Study the drawing (mm; zero at the part's minimum x, y, z) and answer. A direction names the side the tool comes from. Round coordinates to 2 decimals unless told otherwise and drop trailing zeros. Write each loop counter-clockwise with the first axis right and the second up, starting at its lowest first coordinate (ties: lowest second). Pieces come first, ordered by that corner, then holes. Notation, with made-up numbers: (-39, -7.5) - (-9, -7.5) arc R14 ccw to (-9, 4.5) - close; hole circle Ø5 at (23, 80). An arc over 180 degrees is marked (long way). Return JSON: item names as keys, results as strings. Group by question number.
(1) Section B-B, the plane z = 3 is taken. Write down the section's boundary in (x, y), then the cut area to 3 significant figures.
(2) Find the intervals of material crossed by line 1 along X through (y, z) = (48, 18.5); line 2 along Z through (x, y) = (24.5, 19.5); line 3 along X through (y, z) = (5, 9.5) (1 decimal), in increasing order. Write a range as [from, to].
(3) Section C-C, the plane x = 76.2 is taken. Write down the section's boundary in (y, z), then the cut area to 3 significant figures.
(4) Section D-D, the plane y = 57 is taken. Write down the section's boundary in (x, z) (1 decimal).
(5) Each of these flat-tipped pins is pushed along its axis until it touches: pin 1 (2 mm diameter, centred on x = 68.5, z = 23, fed in from +Y); pin 2 (7.5 mm diameter, centred on y = 5.5, z = 9, fed in from -X); pin 3 (4 mm diameter, centred on x = 83.5, z = 4, fed in from -Y); pin 4 (5.5 mm diameter, centred on x = 50.8, y = 75.79, fed in from +Z). Where does it stop, or does it pass through?
(6) Which of the six approach directions +Z, -Z, +X, -X, +Y, -Y give full straight-line access (tool end or side, diameter ignored) to the marked faces 1, 2 and 3?
(7) Section A-A, the plane x = 50.8 is taken. Write down the section's boundary in (y, z) (1 decimal).
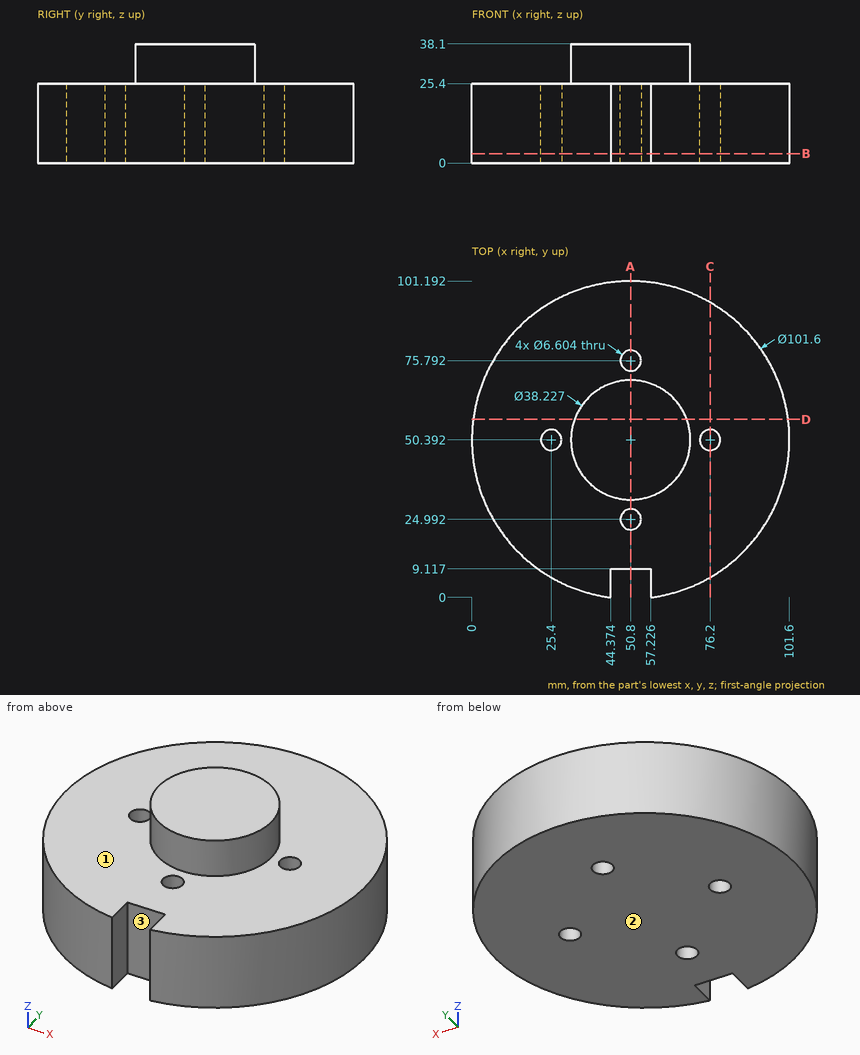
Working result:
{
 "1": {"outline": "(44.37, 0) - (44.37, 9.12) - (57.23, 9.12) - (57.23, 0) arc R50.8 ccw (long way) to start; hole circle Ø6.6 at (25.4, 50.39); hole circle Ø6.6 at (50.8, 24.99); hole circle Ø6.6 at (50.8, 75.79); hole circle Ø6.6 at (76.2, 50.39)", "area": "7,850 mm^2"},
 "2": {"line 1": "x = [0.06, 23.12], [27.68, 73.92], [78.48, 101.54]", "line 2": "z = [0, 25.4]", "line 3": "x = [28, 44.4], [57.2, 73.6]"},
 "3": {"outline": "(6.4, 0) - (47.09, 0) - (47.09, 25.4) - (6.4, 25.4) - close; (53.69, 0) - (94.39, 0) - (94.39, 25.4) - (53.69, 25.4) - close", "area": "2,070 mm^2"},
 "4": {"outline": "(0.4, 0) - (101.2, 0) - (101.2, 25.4) - (68.7, 25.4) - (68.7, 38.1) - (32.9, 38.1) - (32.9, 25.4) - (0.4, 25.4) - close"},
 "5": {"pin 1": "stops at y = 98.37", "pin 2": "stops at x = 21", "pin 3": "stops at y = 9.92", "pin 4": "passes through"},
 "6": {"face 1": "+Z", "face 2": "-Z, +X, -X, +Y, -Y", "face 3": "+Z, -Z, -Y"},
 "7": {"outline": "(9.1, 0) - (21.7, 0) - (21.7, 25.4) - (9.1, 25.4) - close; (28.3, 0) - (72.5, 0) - (72.5, 25.4) - (69.5, 25.4) - (69.5, 38.1) - (31.3, 38.1) - (31.3, 25.4) - (28.3, 25.4) - close; (79.1, 0) - (101.2, 0) - (101.2, 25.4) - (79.1, 25.4) - close"}
}
